```python
from build123d import *

# Parameters (mm, degrees)
F_01_START                = -3
S01_HEAD_R                = 2.75
F_01_HEAD_DEPTH           = 3
S02_NOMINAL_SHANK_R       = 1.5
F_02_NOMINAL_SHANK_DEPTH  = 30
F_03_START                = -3.1
F_03_HEX_KEY_SOCKET_DEPTH = 1.75


with BuildPart() as part:
    # S01 - Head → 01 - Head (new body)
    with BuildSketch(Plane.XY.offset(F_01_START)):
        Circle(S01_HEAD_R)
    extrude(amount=F_01_HEAD_DEPTH)

    # S02 - Nominal shank → 02 - Nominal shank (add)
    with BuildSketch(Plane.XY):
        Circle(S02_NOMINAL_SHANK_R)
    extrude(amount=F_02_NOMINAL_SHANK_DEPTH)

    # S03 - Hex key socket → 03 - Hex key socket (cut)
    with BuildSketch(Plane.XY.offset(F_03_START)):
        Polygon((1.443375673, 0), (0.721687836, 1.25), (-0.721687836, 1.25), (-1.443375673, 0), (-0.721687836, -1.25), (0.721687836, -1.25), align=None)
    extrude(amount=F_03_HEX_KEY_SOCKET_DEPTH, mode=Mode.SUBTRACT)


solid = part.part
```
Design review of the part built by this model. Coordinates are the model's own, in mm. A direction names the side the tool comes from. Round coordinates to 2 decimals unless told otherwise and drop trailing zeros. Order: outer loops, then holes, each group sorted by start corner. A loop starts at its lowest first (then second) coordinate and runs counter-clockwise, first axis right, second up. Notation, with made-up numbers: M 7,-20 L 19,-20 A26 cw 19,14 Z; hole C 12.5,11.25 d8. An arc over 180 degrees is marked long. Put each result on its own line as item: value.
Q1. Insertion check: pin 1 Ø3 at (x, y) = (1, 0) entering from -Z; pin 2 Ø1 at (y, z) = (0, 21) entering from +X; pin 3 Ø3 at (x, z) = (0, 7) entering from -Y. Each pin has a flat end and moves straight along its axis. Give the tip position at first contact, or say it passes through.
Reported:
pin 1: z = -3
pin 2: x = 1.5
pin 3: y = -1.5
Q2. Consider section C-C (z = 0.5). State the section outline as (x, y) points, and give its area (3 significant figures).
Reported:
outline: C 0,0 d3
area: 7.07 mm²
Q3. To check wall thickness, follow line 1 (Z direction, x = 0.45, y = -1); line 2 (X direction, y = 0.4, z = 13); line 3 (Y direction, x = 0.1, z = 9.5). State the ranges of each line that lie inside material, in increasing order.
Reported:
line 1: -1.35 to 30
line 2: -1.45 to 1.45
line 3: -1.5 to 1.5
Q4. Machinability: for faces 5 (the face through (1.2, -1.2, 0)), 6 (the face through (-1.088, -0.616, -2.187)), 7 (the face through (0, 0, 30)), which of the approach directions +Z, -Z, +X, -X, +Y, -Y give a long, thin tool a straight path to every point of the face, cutting with its end or side? Answer none if there is none.
Reported:
face 5: +Z
face 6: -Z
face 7: +Z, +X, -X, +Y, -Y
Q5. Consider section B-B (y = 0.3). State the section outline as (x, z) points.
Reported:
outline: M -2.73,-3 L -1.27,-3 L -1.27,-1.35 L 1.27,-1.35 L 1.27,-3 L 2.73,-3 L 2.73,0 L 1.47,0 L 1.47,30 L -1.47,30 L -1.47,0 L -2.73,0 Z
Q6. Consider section A-A (x = 0). State the section outline as (y, z) points.
Reported:
outline: M -2.75,-3 L -1.25,-3 L -1.25,-1.35 L 1.25,-1.35 L 1.25,-3 L 2.75,-3 L 2.75,0 L 1.5,0 L 1.5,30 L -1.5,30 L -1.5,0 L -2.75,0 Z
Q7. Consider section D-D (x = 1.8). State the section outline as (y, z) points, and give its area (3 significant figures).
Reported:
outline: M -2.08,-3 L 2.08,-3 L 2.08,0 L -2.08,0 Z
area: 12.5 mm²
Q8. Draft analysis for pull direction Y (two halves, no side actions). For faces 1 (the face through (-1.3, -0.6, -3)), 2 (the face through (-0.596, -2.685, -1.521)), 3 (the face through (0, 1.25, -2)), 4 (the face through (-1.08, 0.63, -2.19)), state which applies: released by +Y, released by -Y, zero draft, split by the parting line, or undercut.
Reported:
face 1: zero draft
face 2: split by the parting line
face 3: undercut
face 4: undercut
